```python
from build123d import *

# Parameters (mm, degrees)
F3_W = 2
F3_H = 11
F1_R = 1.6


with BuildPart() as f0:
    # F3 (on Front) → F0 (revolve)
    with BuildSketch(Plane.XZ):
        with Locations((3.5, 5.5)):
            Rectangle(F3_W, F3_H)
    revolve(axis=Axis((0, 0, 71.798525), (0, 0, 1)))

    # F1 (on Front) → F2 (revolve)
    with BuildSketch(Plane.XZ):
        with Locations((5.11, 3.25)):
            Circle(F1_R)
    revolve(axis=Axis((0, 0, 0), (0, 0, 1)))


solid = f0.part
```
CAD build for the part. Positions are in the model's coordinates, mm. A direction names the side the tool comes from. Give positions to 0.01 mm unless a question says otherwise; leave off trailing zeros. Order: outer loops, then holes, each group sorted by start corner. A loop starts at its lowest first (then second) coordinate and runs counter-clockwise, first axis right, second up. Notation, with made-up numbers: M -1.5,10 L 43.5,10 A24 cw 43.5,26 Z; hole C 7.25,76.5 d5. An arc over 180 degrees is marked long. Put each result on its own line as item: value. Start each with the question number.
(1) Saw through at D-D, the plane z = 3.5. Write the cut outline in (x, y).
(2) Saw through at A-A, the plane y = 0. Write the cut outline in (x, z).
(3) Flat gauge pin, fed straight in: pin 1 Ø4 at (x, z) = (3.5, 9.5) entering from -Y. Where does the tip first touch, or does it go through?
(4) Which spindle directions (+Z, -Z, +X, -X, +Y, -Y) get a long thin tool onto all of the face, cutting with end or side? Do faces 1 (the cylindrical face through (-0.59, 4.46, 0.9)), 2 (the flat face through (-2, -2, 0)), 3 (the cylindrical face through (-0.59, 4.46, 7.91)). Say none if no direction does.
(5) Drill centre lines: line 1 along Y through (x, z) = (0, 8.25); line 2 along X through (y, z) = (2.25, 5.5); line 3 along Y through (x, z) = (0, 3). Where is each one in solid material? Low to high.
(6) Saw through at C-C, the plane z = 10. Write the cut outline in (x, y), then the cut area to 3 significant figures.
(7) Mould opens along Y. For faces 4 (the cylindrical face through (-0.54, -2.44, 5.58)), 5 (the flat face through (-2, -2, 11)) say: +Y half, -Y half, draft (parallel to the pull), parting line (faces both ways), or undercut.
Check result:
1. outline: C 0,0 d13.38; hole C 0,0 d5
2. outline: M -4.5,0 L -2.5,0 L -2.5,11 L -4.5,11 L -4.5,4.73 A1.6 ccw long -4.5,1.77 Z; M 2.5,0 L 4.5,0 L 4.5,1.77 A1.6 ccw long 4.5,4.73 L 4.5,11 L 2.5,11 Z
3. pin 1: stops at y = -4.24
4. face 1: -Z
4. face 2: -Z, +X, -X, +Y, -Y
4. face 3: +Z
5. line 1: y = -4.5 to -2.5, 2.5 to 4.5
5. line 2: x = -3.9 to -1.09, 1.09 to 3.9
5. line 3: y = -6.69 to -2.5, 2.5 to 6.69
6. outline: C 0,0 d9; hole C 0,0 d5
6. area: 44.0 mm2
7. face 4: undercut
7. face 5: draft
